Source: CAD feature listing. Evaluate the final solid. Frame: model axes, mm. Face numbers are marked on the shaded views. A direction names the side the tool comes from. Give positions to 0.01 mm unless a question says otherwise; leave off trailing zeros. Order: outer loops, then holes, each group sorted by start corner. A loop starts at its lowest first (then second) coordinate and runs counter-clockwise, first axis right, second up. Notation, with made-up numbers: M 82.25,53 L 87.25,53 A23 cw 87.25,64 Z; hole C 40.25,-13.5 d9. An arc over 180 degrees is marked long. Answer as a JSON object with one key per item and string values. Group by question number.
1. Pin query (flat end, axial travel): P1, Ø3, axis at x = 8, z = 2, coming from the +Y side; P2, Ø6, axis at y = 4.5, z = -3, coming from the -X side; P3, Ø3, axis at x = -5, z = 1, coming from the +Y side; P4, Ø2, axis at y = 16, z = 0.5, coming from the +X side. Return the tip coordinate at first contact, or that it passes through.
2. Section query B-B (y = 24.5). Output: boundary loops of the cut face in (x, z), plus the area to 3 significant figures.
3. Set-up query: the marked faces 1, 2, 3, 4 and 5. Return all of +Z, -Z, +X, -X, +Y, -Y with unobstructed straight access to the full face (end or side cutting, diameter ignored); none if empty.
4. Material intervals for L1, parallel to Y at x = -11, z = 2.75; L2, parallel to X at y = 3, z = -0.5; L3, parallel to Y at x = 10, z = 2, sorted ascending. Write a range as [from, to].
5. Section query C-C (x = 7). Output: boundary loops of the cut face in (y, z).
from build123d import *

# Parameters (mm, degrees)
SKETCH1_W           = 22.225
SKETCH1_H           = 11.1125
BOSS_EXTRUDE1_DEPTH = 23.8125
SKETCH2_W           = 11.1125
SKETCH2_H           = 1.5875
BOSS_EXTRUDE2_DEPTH = 4.7625
SKETCH3_R           = 5.55625
BOSS_EXTRUDE3_DEPTH = 3.175
SKETCH4_R           = 2.38125
BOSS_EXTRUDE4_DEPTH = 3.175


with BuildPart() as part:
    # Sketch1 → Boss-Extrude1 (new body)
    with BuildSketch(Plane(origin=(0, 0, 0), x_dir=(1, 0, 0), z_dir=(0, 1, 0))):
        Rectangle(SKETCH1_W, SKETCH1_H)
    extrude(amount=BOSS_EXTRUDE1_DEPTH)

    # Sketch2 → Boss-Extrude2 (add)
    with BuildSketch(Plane(origin=(11.1125, 0, 0), x_dir=(0, 0, -1), z_dir=(1, 0, 0))):
        with Locations((0, 19.84375)):
            Rectangle(SKETCH2_W, SKETCH2_H)
    boss_extrude2 = extrude(amount=BOSS_EXTRUDE2_DEPTH)

    # Mirror2: Boss-Extrude2 across plane
    add(boss_extrude2.mirror(Plane.ZY))

    # Sketch3 → Boss-Extrude3 (add)
    with BuildSketch(Plane(origin=(0, 23.8125, 0), x_dir=(1, 0, 0), z_dir=(0, 1, 0))):
        with Locations(Location((5.55625, 0, 0), (0, 0, 270))):
            Circle(SKETCH3_R)
    extrude(amount=BOSS_EXTRUDE3_DEPTH)

    # Sketch4 → Boss-Extrude4 (add)
    with BuildSketch(Plane(origin=(0, 26.9875, 0), x_dir=(1, 0, 0), z_dir=(0, 1, 0))):
        with Locations(Location((5.55625, 0, 0), (0, 0, 270))):
            Circle(SKETCH4_R)
    extrude(amount=BOSS_EXTRUDE4_DEPTH)


solid = part.part
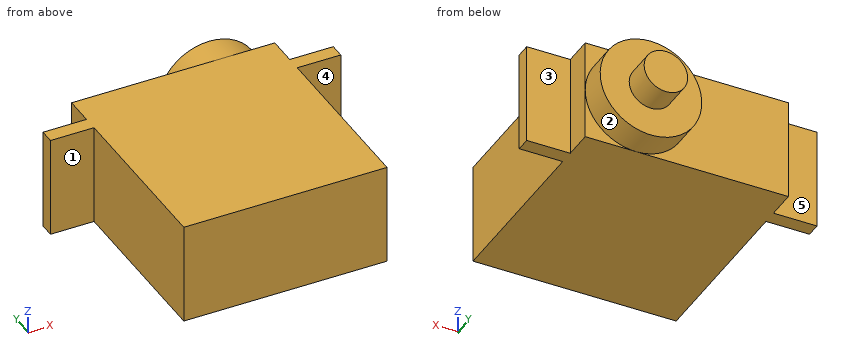
Answer sheet:
{
 "1": {"P1": "y = 30.16", "P2": "x = -11.11", "P3": "y = 23.81", "P4": "x = 11.11"},
 "2": {"outline": "C 5.56,0 d11.11", "area": "97.0 mm^2"},
 "3": {"face 1": "+Z, -Z, -X, -Y", "face 2": "+Y", "face 3": "+Z, -Z, +X, +Y", "face 4": "+Z, -Z, +X, -Y", "face 5": "+Z, -Z, -X, +Y"},
 "4": {"L1": "[0, 23.81]", "L2": "[-11.11, 11.11]", "L3": "[0, 26.99]"},
 "5": {"outline": "M 0,-5.56 L 23.81,-5.56 L 23.81,-5.37 L 26.99,-5.37 L 26.99,-1.89 L 30.16,-1.89 L 30.16,1.89 L 26.99,1.89 L 26.99,5.37 L 23.81,5.37 L 23.81,5.56 L 0,5.56 Z"}
}
